```python
from build123d import *

# Parameters (mm, degrees)
F0_W     = 169.8625
F0_H     = 100
F1_DEPTH = 4.7625
F3_DEPTH = 50
F4_DEPTH = 50
F5_W     = 56
F5_H     = 56
F6_DEPTH = 7.9385


with BuildPart() as f1:
    # F0 (on Top) → F1 (new body)
    with BuildSketch(Plane.XY):
        Rectangle(F0_W, F0_H)
    extrude(amount=F1_DEPTH)

    # F2 (on Right) → F3 (join)
    with BuildSketch(Plane.YZ):
        Polygon((-50, 4.7625), (50, 4.7625), (50, 7.9375), align=None)
    extrude(amount=F3_DEPTH)

    # F3_face (on face) → F4 (join)
    with BuildSketch(Plane(origin=(0, 16.666667, 5.820833), x_dir=(0, 1, 0), z_dir=(-1, 0, 0))):
        Polygon((33.333333, 1.058333), (-66.666667, 1.058333), (33.333333, -2.116667), align=None)
    extrude(amount=F4_DEPTH)

    # F5 (on face) → F6 (cut, through all)
    with BuildSketch(Plane(origin=(0, 0, 0), x_dir=(1, 0, 0), z_dir=(0, 0, -1))):
        Rectangle(F5_W, F5_H)
    extrude(amount=-F6_DEPTH, mode=Mode.SUBTRACT)


solid = f1.part
```
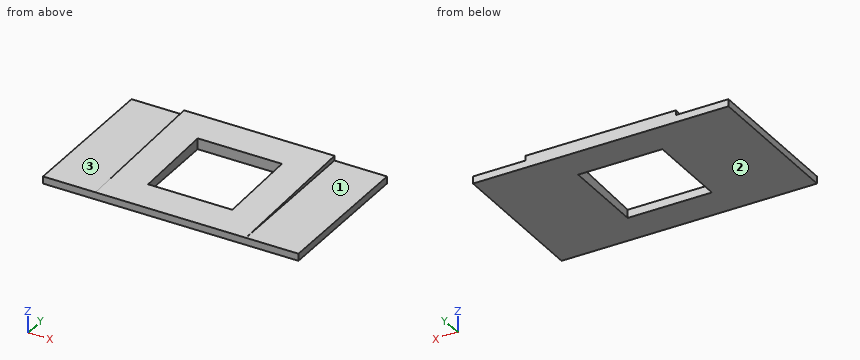
Can you work these out from the model? Positions are in its coordinate system, mm. Face numbers are marked on the shaded views. A direction names the side the tool comes from. Give positions to 0.01 mm unless a question says otherwise; leave off trailing zeros. Loops run counter-clockwise (first coordinate to the right, second up) from the corner with the lowest first, then second, coordinate; pieces in that order, holes last. Notation, with made-up numbers: M 74.5,37.5 L 89.5,37.5 A25 cw 89.5,61.5 Z; hole C -11,30.5 d5. An arc over 180 degrees is marked long. Use one line per item in the form item = value. Start each with the question number.
(1) I want a section at C-C, the plane z = 3. Write out the boundary of the cut face in (x, y).
(2) I'm going to push flat-ended pins straight in: P1, Ø1, axis at x = -63.5, y = 1.5, coming from the -Z side; P2, Ø1.5, axis at x = 9, z = 7, coming from the -Y side. Where does each tip first touch, or does it pass through?
(3) On a 3-axis mill with a long thin cutter (end or side, diameter ignored), from which of +Z, -Z, +X, -X, +Y, -Y can I reach the whole of each face in a straight line? I mean the marked faces 1, 2 and 3. Say none if no direction works.
(4) I want a section at B-B, the plane y = 10. Write out the boundary of the cut face in (x, z).
(5) I want a section at D-D, the plane y = -35.5. Write out the boundary of the cut face in (x, z).
(6) Please list where these lines run through material, in increasing order: line 1 (Y direction, x = -10, z = 3.25); line 2 (X direction, y = -18, z = 2.75).
(7) I want a section at A-A, the plane x = 16.5. Write out the boundary of the cut face in (y, z), and give its area (3 significant figures).
Worked out:
q1.outline = M -84.93,-50 L 84.93,-50 L 84.93,50 L -84.93,50 Z; hole M -28,-28 L 28,-28 L 28,28 L -28,28 Z
q2.P1 = 0
q2.P2 = 28
q3.face_1 = +Z, +X, +Y, -Y
q3.face_2 = -Z, +X, -X, +Y, -Y
q3.face_3 = +Z, -X, +Y, -Y
q4.outline = M -84.93,0 L -28,0 L -28,6.67 L -50,6.67 L -50,4.76 L -84.93,4.76 Z; M 28,0 L 84.93,0 L 84.93,4.76 L 50,4.76 L 50,6.67 L 28,6.67 Z
q5.outline = M -84.93,0 L 84.93,0 L 84.93,4.76 L 50,4.76 L 50,5.22 L -50,5.22 L -50,4.76 L -84.93,4.76 Z
q6.line_1 = -50 to -28, 28 to 50
q6.line_2 = -84.93 to -28, 28 to 84.93
q7.outline = M -50,0 L -28,0 L -28,5.46 L -50,4.76 Z; M 28,0 L 50,0 L 50,7.94 L 28,7.24 Z
q7.area = 279 mm²
